Design review of the part shown in the three views and the two pictorial views. Dimensions are in mm from the part's minimum x, y and z. Round coordinates to 2 decimals unless told otherwise and drop trailing zeros. Order: outer loops, then holes, each group sorted by start corner. A loop starts at its lowest first (then second) coordinate and runs counter-clockwise, first axis right, second up.
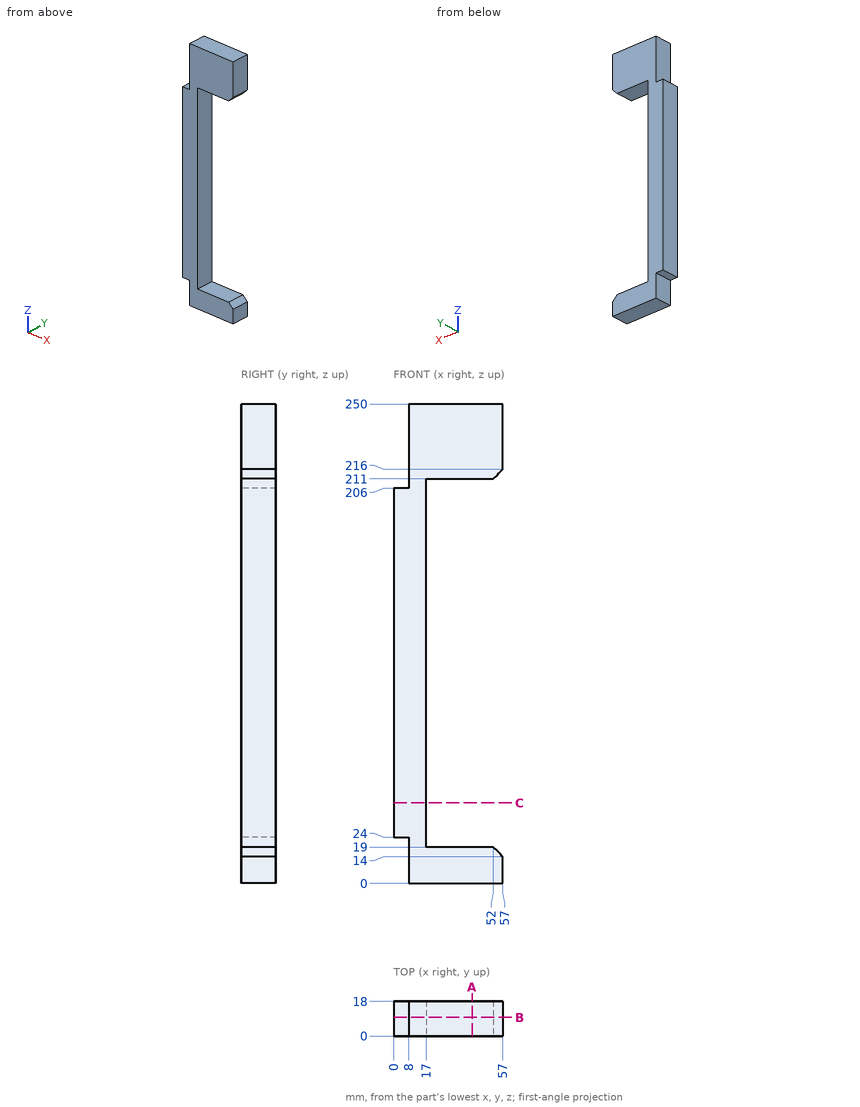
1) Take a section at A-A on x = 41. Give the boundary of the cut face in (y, z), plus the area to 3 significant figures.
Results:
outline: (0, 0) - (18, 0) - (18, 19) - (0, 19) - close; (0, 211) - (18, 211) - (18, 250) - (0, 250) - close
area: 1,040 mm2
2) Clearance check with flat-ended pins moving along their axes: P1, Ø5.5, axis at y = 9.5, z = 236, coming from the -X side; P2, Ø4, axis at y = 3, z = 35, coming from the +X side; P3, Ø8, axis at x = 23.5, z = 117, coming from the +Y side; P4, Ø9, axis at x = 3, y = 7, coming from the -Z side. State where each tip first meets the part, or that it passes through.
Results:
P1: stops at x = 8
P2: stops at x = 17
P3: passes through
P4: stops at z = 24
3) Take a section at B-B on y = 9.75. Give the boundary of the cut face in (x, z).
Results:
outline: (0, 24) - (8, 24) - (8, 0) - (57, 0) - (57, 14) - (52, 19) - (17, 19) - (17, 211) - (52, 211) - (57, 216) - (57, 250) - (8, 250) - (8, 206) - (0, 206) - close
4) Take a section at C-C on z = 42. Give the boundary of the cut face in (x, y), plus the area to 3 significant figures.
Results:
outline: (0, 0) - (17, 0) - (17, 18) - (0, 18) - close
area: 306 mm2
5) To check wall thickness, follow line 1 along Z through (x, y) = (51.5, 11.75); line 2 along X through (y, z) = (17, 182.5); line 3 along Z through (x, y) = (2, 1.5). State the ranges of each line that lie inside material, in increasing order.
Results:
line 1: z = 0 to 19, 211 to 250
line 2: x = 0 to 17
line 3: z = 24 to 206
